```python
from build123d import *

# Parameters (mm, degrees)
EXTRUDE_1_DEPTH          = 40
SKETCH_4_W               = 52
SKETCH_4_H               = 10
CUT_EXTRUDE_1_DEPTH      = 8
SKETCH_7_W               = 52
SKETCH_7_H               = 10
CUT_EXTRUDE_2_DEPTH      = 8
CUT_EXTRUDE_3_DEPTH      = 67.792933004
CUT_EXTRUDE_3_DEPTH_BACK = 67.792933004


with BuildPart() as part:
    # 草圖2 → 填料-伸長1 (new body)
    with BuildSketch(Plane.XY):
        with BuildLine():
            Line((0, 0), (52, 0))
            Line((52, 0), (52, 22))
            Line((52, 22), (9.683462586, 64.316537414))
            Line((9.683462586, 64.316537414), (-1.630245913, 64.316537414))
            Line((-1.630245913, 64.316537414), (33.857864376, 28.828427125))
            ThreePointArc((33.857864376, 28.828427125), (34.724955382, 24.469266271), (31.029437252, 22))
            Line((31.029437252, 22), (0, 22))
            Line((0, 22), (0, 0))
        make_face()
    extrude(amount=-EXTRUDE_1_DEPTH)

    # 草圖4 → 除料-伸長1 (cut)
    with BuildSketch(Plane.XY):
        with Locations((26, 5)):
            Rectangle(SKETCH_4_W, SKETCH_4_H)
    extrude(amount=-CUT_EXTRUDE_1_DEPTH, mode=Mode.SUBTRACT)

    # 草圖7 → 除料-伸長2 (cut)
    with BuildSketch(Plane(origin=(0, 0, -40), x_dir=(-1, 0, 0), z_dir=(0, 0, -1))):
        with Locations((-26, 5)):
            Rectangle(SKETCH_7_W, SKETCH_7_H)
    extrude(amount=-CUT_EXTRUDE_2_DEPTH, mode=Mode.SUBTRACT)

    # 草圖9 → 除料-伸長3 (cut, two sides: drawn at the far end of the back side and taken through both)
    with BuildSketch(Plane(origin=(37, 37, 0), x_dir=(0, 0, -1), z_dir=(0.7071067811865432, 0.7071067811865519, 0)).offset(-CUT_EXTRUDE_3_DEPTH_BACK)):
        Polygon((12, 232.582795613), (12, 46.631417687), (12, 34.631417687), (20, 26.631417687), (28, 34.631417687), (28, 46.631417687), (28, 232.582795613), (28, 604.485551465), (12, 604.485551465), align=None)
    extrude(amount=CUT_EXTRUDE_3_DEPTH + CUT_EXTRUDE_3_DEPTH_BACK, mode=Mode.SUBTRACT)


solid = part.part
```
Build history of the part. All positions in model axes, mm. A direction names the side the tool comes from. Round coordinates to 2 decimals unless told otherwise and drop trailing zeros. Order: outer loops, then holes, each group sorted by start corner. A loop starts at its lowest first (then second) coordinate and runs counter-clockwise, first axis right, second up. Notation, with made-up numbers: (18, 42) - (68, 42) arc R25 ccw to (68, 70) - close; hole circle Ø8 at (54, 57.25). An arc over 180 degrees is marked (long way). Use a Markdown table: item, result.
1) Wall check: L1, parallel to X at y = 17.5, z = -33; L2, parallel to Y at x = 10.5, z = -21.5; L3, parallel to Y at x = 15, z = -34.5. Give the ranges that are in metal, low to high.
Recorded:
| item | result |
|---|---|
| L1 | x = 0 to 52 |
| L2 | y = 0 to 22 |
| L3 | y = 10 to 22, 47.69 to 59 |
2) Saw through at A-A on z = -33. Write the cut outline in (x, y).
Recorded:
| item | result |
|---|---|
| outline | (-1.63, 64.32) - (33.86, 28.83) arc R4 cw to (31.03, 22) - (0, 22) - (0, 10) - (52, 10) - (52, 22) - (9.68, 64.32) - close |
3) Pull direction Y, two halves, no side cores. Call faces 1 (the face through (26, 10, -4)), 2 (the face through (6, 61, -28)), 3 (the face through (15.865, 46.821, -19.72)), 4 (the face through (34.75, 24.53, -19.72)): pulls with the +Y half, pulls with the -Y half, needs draft (parallel to the pull), parting line crosses it, or undercut.
Recorded:
| item | result |
|---|---|
| face 1 | pulls with the -Y half |
| face 2 | needs draft |
| face 3 | undercut |
| face 4 | undercut |
4) Saw through at B-B on x = 6. Write the cut outline in (y, z).
Recorded:
| item | result |
|---|---|
| outline | (0, -32) - (10, -32) - (10, -40) - (22, -40) - (22, 0) - (10, 0) - (10, -8) - (0, -8) - close; (56.69, -40) - (64.32, -40) - (64.32, -28) - (56.69, -28) - close; (56.69, -12) - (64.32, -12) - (64.32, 0) - (56.69, 0) - close |
5) Tool access for faces 5 (the face through (26, 5, -32)), 6 (the face through (6, 61, -12)), 7 (the face through (16, 22, -20)), 8 (the face through (26, 5, -8)): list every direction of +Z, -Z, +X, -X, +Y, -Y with a clear straight run to the whole face (end or side of a thin tool).
Recorded:
| item | result |
|---|---|
| face 5 | -Z, +X, -X, -Y |
| face 6 | -X, +Y |
| face 7 | +Z, -Z, -X |
| face 8 | +Z, +X, -X, -Y |
6) Flat gauge pins, fed straight in: pin 1 Ø3 at (x, y) = (13, 3.5) entering from -Z; pin 2 Ø4 at (x, y) = (22.5, 56) entering from -Z; pin 3 Ø11 at (x, y) = (35.5, 3) entering from +Z; pin 4 Ø5 at (y, z) = (28.5, -24) entering from +X. Where does each tip first touch, or does it go through?
Recorded:
| item | result |
|---|---|
| pin 1 | stops at z = -32 |
| pin 2 | passes through |
| pin 3 | stops at z = -8 |
| pin 4 | stops at x = 48 |
7) Saw through at D-D on y = 58. Write the cut outline in (x, z).
Recorded:
| item | result |
|---|---|
| outline | (4.69, -40) - (16, -40) - (16, -23.07) - (9.02, -28) - (4.69, -28) - close; (4.69, -12) - (9.02, -12) - (16, -16.93) - (16, 0) - (4.69, 0) - close |
8) Saw through at C-C on x = 38. Write the cut outline in (y, z).
Recorded:
| item | result |
|---|---|
| outline | (0, -32) - (10, -32) - (10, -40) - (36, -40) - (36, 0) - (10, 0) - (10, -8) - (0, -8) - close |
